CAD build for the part. Positions are in the model's coordinates, mm. A direction names the side the tool comes from. Give positions to 0.01 mm unless a question says otherwise; leave off trailing zeros. Loops run counter-clockwise (first coordinate to the right, second up) from the corner with the lowest first, then second, coordinate; pieces in that order, holes last.
```python
from build123d import *

# Parameters (mm, degrees)
SKETCH_1_W            = 20
SKETCH_1_H            = 15
EXTRUDE_1_DEPTH       = 10
F_3_0MM_1_D           = 3
F_3_0MM_1_CSINK_D     = 3.05
F_3_0MM_1_CSINK_ANGLE = 90
SKETCH_3_W            = 20
SKETCH_3_H            = 26
EXTRUDE_2_DEPTH       = 3
F_2_5MM_1_D           = 2.5
F_2_5MM_1_CSINK_D     = 2.55
F_2_5MM_1_CSINK_ANGLE = 90
CHAMFER_1_SIZE        = 2


with BuildPart() as part:
    # 草图1 → 凸台-拉伸1 (new body)
    with BuildSketch(Plane.XY):
        with Locations((10, 7.5)):
            Rectangle(SKETCH_1_W, SKETCH_1_H)
    extrude(amount=EXTRUDE_1_DEPTH)

    # Ø3.0mm 暗销孔1 (through all)
    with Locations(Plane(origin=(4, 11, 10), x_dir=(1, 0, 0), z_dir=(0, 0, 1))):
        with Locations((0, 0), (12, 0)):
            CounterSinkHole(F_3_0MM_1_D / 2, F_3_0MM_1_CSINK_D / 2, counter_sink_angle=F_3_0MM_1_CSINK_ANGLE)

    # 草图3 → 凸台-拉伸2 (add)
    with BuildSketch(Plane.XZ):
        with Locations((10, 5)):
            Rectangle(SKETCH_3_W, SKETCH_3_H)
    extrude(amount=EXTRUDE_2_DEPTH)

    # Ø2.5mm 暗销孔1 (through all)
    with Locations(Plane(origin=(5, -3, 13), x_dir=(0, 0, -1), z_dir=(0, -1, 0))):
        with Locations((0, 0), (0, 10), (16, 0), (16, 10)):
            CounterSinkHole(F_2_5MM_1_D / 2, F_2_5MM_1_CSINK_D / 2, counter_sink_angle=F_2_5MM_1_CSINK_ANGLE)

    # 倒角1
    chamfer_1_edges = [part.edges().sort_by_distance(p)[0] for p in [
        (20, -1.5, -8),
        (20, -1.5, 18),
        (0, -1.5, 18),
        (0, -1.5, -8),
    ]]
    chamfer(chamfer_1_edges, length=CHAMFER_1_SIZE)


solid = part.part
```
1. Drop flat-ended pins along their axis: pin 1 (4 mm diameter, centred on x = 16, y = 11, fed in from -Z); pin 2 (3.5 mm diameter, centred on x = 4, y = 11, fed in from +Z); pin 3 (3 mm diameter, centred on x = 5, z = 13, fed in from +Y). Give the stop position or say it passes through.
Responses:
pin 1: stops at z = 0
pin 2: stops at z = 10
pin 3: stops at y = 0
2. Probe line 1 along X through (y, z) = (11, 7.25); line 2 along X through (y, z) = (-1.15, 13); line 3 along Z through (x, y) = (15, -1.4). List the from-to ranges inside material, lowest first.
Responses:
line 1: x = 0 to 2.5, 5.5 to 14.5, 17.5 to 20
line 2: x = 0 to 3.75, 6.25 to 13.75, 16.25 to 20
line 3: z = -8 to -4.25, -1.75 to 11.75, 14.25 to 18
3. Saw through at D-D, the plane x = 5. Count the separate pieces of the cut face and the enclosed holes in it, and give its area (3 significant figures).
Responses:
separate pieces: 4
enclosed holes: 0
area: 191 mm2
4. Tool access for faces 1 (the face through (2.614, 10.425, 4.918)), 2 (the face through (10, 0, 14)), 3 (the face through (10, 8, 0)): list every direction of +Z, -Z, +X, -X, +Y, -Y with a clear straight run to the whole face (end or side of a thin tool).
Responses:
face 1: +Z, -Z
face 2: +Z, +X, -X, +Y
face 3: -Z, +X, -X, +Y
5. Saw through at C-C, the plane z = 4.25. List the corners of the cut face in (x, y), and give its area (3 significant figures).
Responses:
outline: (0, -3) - (20, -3) - (20, 15) - (0, 15) - close; hole circle Ø3 at (4, 11); hole circle Ø3 at (16, 11)
area: 346 mm2
6. Saw through at B-B, the plane z = -3. List the corners of the cut face in (x, y) (3 decimals), and give its area (3 significant figures).
Responses:
outline: (0, -3) - (3.725, -3) - (3.75, -2.975) - (3.75, 0) - (0, 0) - close; (6.25, -2.975) - (6.275, -3) - (13.725, -3) - (13.75, -2.975) - (13.75, 0) - (6.25, 0) - close; (16.25, -2.975) - (16.275, -3) - (20, -3) - (20, 0) - (16.25, 0) - close
area: 45.0 mm2
7. Saw through at A-A, the plane y = 11. List the corners of the cut face in (x, z) (3 decimals), and give its area (3 significant figures).
Responses:
outline: (0, 0) - (2.5, 0) - (2.5, 9.975) - (2.475, 10) - (0, 10) - close; (5.5, 0) - (14.5, 0) - (14.5, 9.975) - (14.475, 10) - (5.525, 10) - (5.5, 9.975) - close; (17.5, 0) - (20, 0) - (20, 10) - (17.525, 10) - (17.5, 9.975) - close
area: 140 mm2
8. Pull direction X, two halves, no side cores. Call faces 4 (the face through (10, 8, 10)), 5 (the face through (20, 6, 5)), 6 (the face through (3.891, -1.467, -2.423)), 7 (the face through (1, -1, 17)): released by +X, released by -X, zero draft, split by the parting line, or undercut.
Responses:
face 4: zero draft
face 5: released by +X
face 6: undercut
face 7: released by -X
